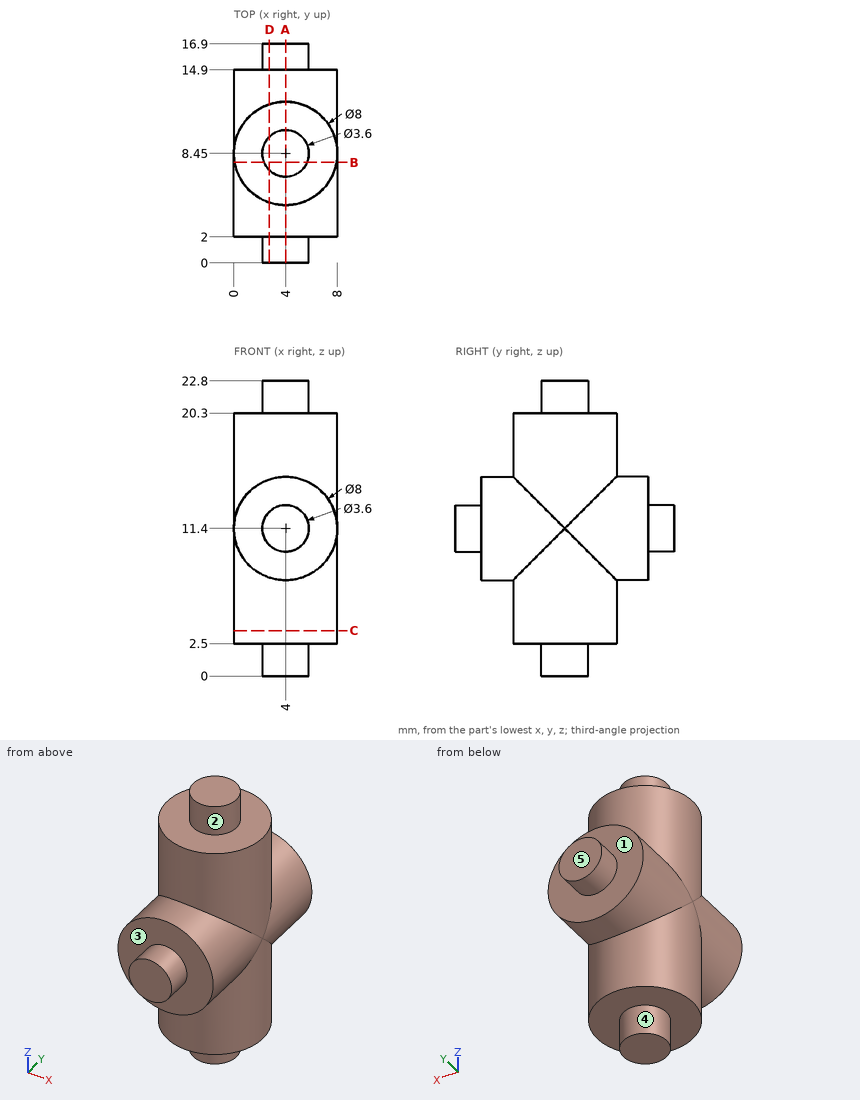
Print and shaded views of the part. All mm, measured from the part's lowest x, y and z. A direction names the side the tool comes from. Give positions to 0.01 mm unless a question says otherwise; leave off trailing zeros. Order: outer loops, then holes, each group sorted by start corner. A loop starts at its lowest first (then second) coordinate and runs counter-clockwise, first axis right, second up. Notation, with made-up numbers: (17.5, 26.25) - (23.5, 26.25) arc R32 cw to (23.5, 60.25) - close; hole circle Ø5 at (25, 80.5). An arc over 180 degrees is marked (long way). Use a Markdown table: item, result.
1) Saw through at D-D on x = 2.75. List the corners of the cut face in (y, z).
Checked values:
| item | result |
|---|---|
| outline | (0, 10.1) - (2, 10.1) - (2, 7.6) - (4.65, 7.6) - (4.65, 2.5) - (7.15, 2.5) - (7.15, 0) - (9.75, 0) - (9.75, 2.5) - (12.25, 2.5) - (12.25, 7.6) - (14.9, 7.6) - (14.9, 10.1) - (16.9, 10.1) - (16.9, 12.7) - (14.9, 12.7) - (14.9, 15.2) - (12.25, 15.2) - (12.25, 20.3) - (9.75, 20.3) - (9.75, 22.8) - (7.15, 22.8) - (7.15, 20.3) - (4.65, 20.3) - (4.65, 15.2) - (2, 15.2) - (2, 12.7) - (0, 12.7) - close |
2) Probe L1, parallel to Y at x = 7, z = 9.25; L2, parallel to Z at x = 5.5, y = 9.5; L3, parallel to Z at x = 6, y = 2.5. List the from-to ranges inside material, lowest first. Write a range as from..to.
Checked values:
| item | result |
|---|---|
| L1 | 2..14.9 |
| L2 | 2.5..20.3 |
| L3 | 7.94..14.86 |
3) Saw through at B-B on y = 7.75. List the corners of the cut face in (x, z).
Checked values:
| item | result |
|---|---|
| outline | (0.06, 2.5) - (2.34, 2.5) - (2.34, 0) - (5.66, 0) - (5.66, 2.5) - (7.94, 2.5) - (7.94, 10.7) arc R4 ccw to (7.94, 12.1) - (7.94, 20.3) - (5.66, 20.3) - (5.66, 22.8) - (2.34, 22.8) - (2.34, 20.3) - (0.06, 20.3) - (0.06, 12.1) arc R4 ccw to (0.06, 10.7) - close |
4) 3-axis set-ups, long thin cutter, end or side, ignore diameter. For the marked faces 1, 2, 3, 4 and 5: which of +Z, -Z, +X, -X, +Y, -Y reach the whole face in a straight line?
Checked values:
| item | result |
|---|---|
| face 1 | +Y |
| face 2 | +Z |
| face 3 | -Y |
| face 4 | -Z |
| face 5 | +Z, -Z, +X, -X, +Y |
5) Flat gauge pins, fed straight in: P1, Ø1, axis at x = 6.5, y = 2.5, coming from the +Z side; P2, Ø6, axis at y = 3, z = 16.5, coming from the +X side; P3, Ø5, axis at y = 13.5, z = 3.5, coming from the +X side. Where does each tip first touch, or does it go through?
Checked values:
| item | result |
|---|---|
| P1 | z = 14.86 |
| P2 | x = 7.4 |
| P3 | x = 7.08 |
6) Saw through at C-C on z = 3.5. List the corners of the cut face in (x, y), plus the area to 3 significant figures.
Checked values:
| item | result |
|---|---|
| outline | circle Ø8 at (4, 8.45) |
| area | 50.3 mm² |
7) Saw through at A-A on x = 4. List the corners of the cut face in (y, z).
Checked values:
| item | result |
|---|---|
| outline | (0, 9.6) - (2, 9.6) - (2, 7.4) - (4.45, 7.4) - (4.45, 2.5) - (6.65, 2.5) - (6.65, 0) - (10.25, 0) - (10.25, 2.5) - (12.45, 2.5) - (12.45, 7.4) - (14.9, 7.4) - (14.9, 9.6) - (16.9, 9.6) - (16.9, 13.2) - (14.9, 13.2) - (14.9, 15.4) - (12.45, 15.4) - (12.45, 20.3) - (10.25, 20.3) - (10.25, 22.8) - (6.65, 22.8) - (6.65, 20.3) - (4.45, 20.3) - (4.45, 15.4) - (2, 15.4) - (2, 13.2) - (0, 13.2) - close |
